Geometry check sheet. Reference: drawing and pictorial views, mm from the part's lowest x, y, z. A direction names the side the tool comes from. Round coordinates to 2 decimals unless told otherwise and drop trailing zeros. Loops run counter-clockwise (first coordinate to the right, second up) from the corner with the lowest first, then second, coordinate; pieces in that order, holes last. Notation, with made-up numbers: (88, -8) - (129, -8) arc R17 ccw to (129, 21) - close; hole circle Ø2 at (87.25, 8.25). An arc over 180 degrees is marked (long way). Return JSON: item names as keys, results as strings.
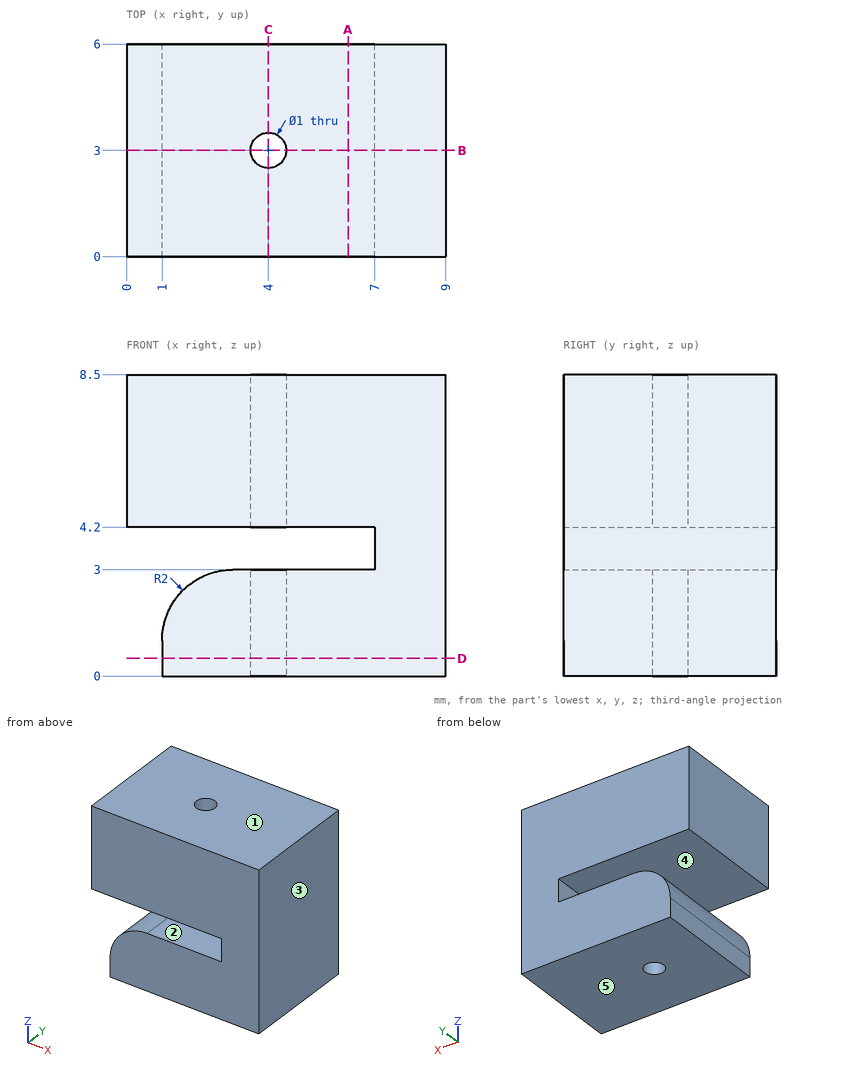
Q1. Sectioned sample at D-D (z = 0.5). Enter the section's corners in (x, y).
Answer key:
{"outline": "(1, 0) - (9, 0) - (9, 6) - (1, 6) - close; hole circle Ø1 at (4, 3)"}
Q2. Sectioned sample at A-A (x = 6.25). Enter the section's corners in (y, z).
Answer key:
{"outline": "(0, 0) - (6, 0) - (6, 3) - (0, 3) - close; (0, 4.2) - (6, 4.2) - (6, 8.5) - (0, 8.5) - close"}
Q3. Sectioned sample at B-B (y = 3). Enter the section's corners in (x, z).
Answer key:
{"outline": "(0, 4.2) - (3.5, 4.2) - (3.5, 8.5) - (0, 8.5) - close; (1, 0) - (3.5, 0) - (3.5, 3) - (3, 3) arc R2 ccw to (1, 1) - close; (4.5, 0) - (9, 0) - (9, 8.5) - (4.5, 8.5) - (4.5, 4.2) - (7, 4.2) - (7, 3) - (4.5, 3) - close"}
Q4. Scan lines: probe 1 along Z at (x, y) = (6.25, 0.95); probe 2 along Y at (x, z) = (4, 6); probe 3 along X at (y, z) = (3.1, 2). Record each from-to range of solid material in increasing order. Write a range as [from, to].
Answer key:
{"probe 1": "z = [0, 3], [4.2, 8.5]", "probe 2": "y = [0, 2.5], [3.5, 6]", "probe 3": "x = [1.27, 3.51], [4.49, 9]"}
Q5. Tool access check on the marked faces 1 and 2. Record the directions out of +Z, -Z, +X, -X, +Y, -Y that give a thin tool (end or side, any length) a straight path to the whole face; none if there is none.
Answer key:
{"face 1": "+Z, +X, -X, +Y, -Y", "face 2": "-X, +Y, -Y"}
Q6. Draft check along Z on the marked faces 3, 4 and 5. Enter one of: released by +Z, released by -Z, zero draft, split by the parting line, or undercut.
Answer key:
{"face 3": "zero draft", "face 4": "undercut", "face 5": "released by -Z"}
Q7. Depth check by flat-ended pin: P1, Ø0.5, axis at y = 4.5, z = 0.5, coming from the -X side. Enter the tip coordinate at first touch or a pass-through.
Answer key:
{"P1": "stops at x = 1"}
Q8. Sectioned sample at C-C (x = 4). Enter the section's corners in (y, z), plus the area to 3 significant figures.
Answer key:
{"outline": "(0, 0) - (2.5, 0) - (2.5, 3) - (0, 3) - close; (0, 4.2) - (2.5, 4.2) - (2.5, 8.5) - (0, 8.5) - close; (3.5, 0) - (6, 0) - (6, 3) - (3.5, 3) - close; (3.5, 4.2) - (6, 4.2) - (6, 8.5) - (3.5, 8.5) - close", "area": "36.5 mm²"}
